```python
from build123d import *

# Parameters (mm, degrees)
SKETCH1_W               = 40
SKETCH1_H               = 55
SKETCH1_H_2             = 20
SKETCH1_R               = 2.5
BOSS_EXTRUDE1_DEPTH     = 10
SKETCH3_W               = 40
SKETCH3_H               = 10
BOSS_EXTRUDE2_DEPTH     = 40
SKETCH4_W               = 9
SKETCH4_H               = 3.5
BOSS_EXTRUDE3_DEPTH     = 40
SKETCH5_R               = 1.5
CUT_EXTRUDE1_DEPTH      = 3.5
SKETCH7_W               = 40
SKETCH7_H               = 3.5
BOSS_EXTRUDE4_DEPTH     = 80
SKETCH8_W               = 12
SKETCH8_H               = 40
BOSS_EXTRUDE5_DEPTH     = 35
SKETCH9_W               = 12
SKETCH9_H               = 23
CUT_EXTRUDE2_DEPTH      = 17
SKETCH10_R              = 1.7
CUT_EXTRUDE3_DEPTH      = 1
CUT_EXTRUDE3_DEPTH_BACK = 38.5
FILLET1_R               = 1
FILLET2_R               = 40


with BuildPart() as part:
    # Sketch1 → Boss-Extrude1 (new body)
    with BuildSketch(Plane(origin=(0, 0, 0), x_dir=(0, 0, -1), z_dir=(1, 0, 0))):
        with Locations((0, 27.5)):
            Rectangle(SKETCH1_W, SKETCH1_H)
        with Locations((0, -10)):
            Rectangle(SKETCH1_W, SKETCH1_H_2)
        with Locations((10, -10)):
            Circle(SKETCH1_R, mode=Mode.SUBTRACT)
        with Locations((-10, -10)):
            Circle(SKETCH1_R, mode=Mode.SUBTRACT)
    extrude(amount=BOSS_EXTRUDE1_DEPTH)

    # Sketch3 → Boss-Extrude2 (add)
    with BuildSketch(Plane.ZY):
        with Locations((0, 5)):
            Rectangle(SKETCH3_W, SKETCH3_H)
    extrude(amount=BOSS_EXTRUDE2_DEPTH)

    # Sketch4 → Boss-Extrude3 (add)
    with BuildSketch(Plane.ZY):
        with Locations((-15.5, 53.25)):
            Rectangle(SKETCH4_W, SKETCH4_H)
    boss_extrude3 = extrude(amount=BOSS_EXTRUDE3_DEPTH)

    # Sketch5 → Cut-Extrude1 (cut)
    with BuildSketch(Plane(origin=(0, 55, 0), x_dir=(1, 0, 0), z_dir=(0, 1, 0))):
        with Locations((-35, 15)):
            Circle(SKETCH5_R)
        with Locations((-4, 15)):
            Circle(SKETCH5_R)
    cut_extrude1 = extrude(amount=-CUT_EXTRUDE1_DEPTH, mode=Mode.SUBTRACT)

    # Mirror2: Boss-Extrude3, Cut-Extrude1 across plane
    add(boss_extrude3.mirror(Plane.XY))
    add(cut_extrude1.mirror(Plane.XY), mode=Mode.SUBTRACT)

    # Sketch7 → Boss-Extrude4 (add)
    with BuildSketch(Plane.XY.offset(20)):
        with Locations((-20, 53.25)):
            Rectangle(SKETCH7_W, SKETCH7_H)
        Polygon((10, 55), (0, 55), (0, 51.5), (0, 25), (10, 25), align=None)
    extrude(amount=BOSS_EXTRUDE4_DEPTH)

    # Sketch8 → Boss-Extrude5 (add)
    with BuildSketch(Plane(origin=(0, 55, 0), x_dir=(1, 0, 0), z_dir=(0, 1, 0))):
        with Locations((-20, -80)):
            Rectangle(SKETCH8_W, SKETCH8_H)
    extrude(amount=BOSS_EXTRUDE5_DEPTH)

    # Sketch9 → Cut-Extrude2 (cut)
    with BuildSketch(Plane(origin=(0, 0, 60), x_dir=(-1, 0, 0), z_dir=(0, 0, -1))):
        with Locations((20, 72.5)):
            Rectangle(SKETCH9_W, SKETCH9_H)
    extrude(amount=-CUT_EXTRUDE2_DEPTH, mode=Mode.SUBTRACT)

    # Sketch10 → Cut-Extrude3 (cut, two sides)
    with BuildSketch(Plane(origin=(0, 90, 0), x_dir=(1, 0, 0), z_dir=(0, 1, 0))) as cut_extrude3_sk:
        with Locations((-20, -68)):
            Circle(SKETCH10_R)
    extrude(amount=CUT_EXTRUDE3_DEPTH, mode=Mode.SUBTRACT)
    extrude(cut_extrude3_sk.sketch, amount=-CUT_EXTRUDE3_DEPTH_BACK, mode=Mode.SUBTRACT)

    # Fillet1
    fillet1_edges = [part.edges().sort_by_distance(p)[0] for p in [
        (-33, 55, 100),
        (-26, 55, 80),
        (-26, 87, 60),
        (-26, 72.5, 100),
        (-14, 55, 80),
        (-14, 72.5, 100),
        (-20, 55, 60),
        (-14, 87, 60),
        (-26, 90, 80),
        (-20, 90, 100),
        (-14, 90, 80),
        (-26, 58, 60),
        (-14, 58, 60),
        (-14, 72.5, 77),
        (-14, 61, 68.5),
        (-20, 84, 77),
        (-14, 84, 68.5),
        (-26, 72.5, 77),
        (-26, 84, 68.5),
        (-20, 61, 77),
        (-26, 61, 68.5),
        (-20, 51.5, 100),
        (0, 38.25, 100),
        (5, 25, 100),
        (10, 40, 100),
        (-2, 55, 100),
        (-40, 53.25, 100),
    ]]
    fillet(fillet1_edges, radius=FILLET1_R)

    # Fillet2
    fillet2_edges = [part.edges().sort_by_distance(p)[0] for p in [
        (5, 25, 20),
    ]]
    fillet(fillet2_edges, radius=FILLET2_R)


solid = part.part
```
Geometry check sheet. Reference: the model listing, model coordinates, mm. A direction names the side the tool comes from. Round coordinates to 2 decimals unless told otherwise and drop trailing zeros. Write each loop counter-clockwise with the first axis right and the second up, starting at its lowest first coordinate (ties: lowest second). Pieces come first, ordered by that corner, then holes. Notation, with made-up numbers: (10, 81) -> (19, 81) arc R7 cw to (19, 88) -> close; hole circle Ø11 at (27, 51). An arc over 180 degrees is marked (long way). Put each result on its own line as item: value.
1) Cross-section at C-C, the plane x = -20. Give the number of separate pieces and of enclosed holes in the cut face, plus the area to 3 significant figures.
Recorded:
separate pieces: 5
enclosed holes: 0
area: 1,750 mm2
2) Cross-section at A-A, the plane x = -9. Enter the section's corners in (y, z).
Recorded:
outline: (0, -20) -> (10, -20) -> (10, 28.78) arc R40 cw to (0, 22.92) -> close; (51.5, -20) -> (55, -20) -> (55, -11) -> (51.5, -11) -> close; (51.5, 11) -> (55, 11) -> (55, 99) arc R1 ccw to (54, 100) -> (52.5, 100) arc R1 ccw to (51.5, 99) -> close
3) Access from +Z, -Z, +X, -X, +Y, -Y to the whole of each face (thin tool, end or side, straight path). Record for faces 5 (the face through (-36.2, 53.3, 14.1)), 6 (the face through (-20, 10, 4)), 7 (the face through (5, 25, 79)), 8 (the face through (-20, 58, 60)), 9 (the face through (-20, 73, 77)).
Recorded:
face 5: +Y
face 6: +Z, -Z, -X
face 7: +Z, +X, -X, -Y
face 8: -Z, +X, -X, +Y
face 9: -Z, +X, -X
4) Cross-section at D-D, the plane z = 3. Enter the section's corners in (x, y), plus the area to 3 significant figures.
Recorded:
outline: (-40, 0) -> (0, 0) -> (0, -20) -> (10, -20) -> (10, 55) -> (0, 55) -> (0, 10) -> (-40, 10) -> close
area: 1,150 mm2
5) Thickness scan on probe 1 along X at (y, z) = (52, -15); probe 2 along X at (y, z) = (88, 68); probe 3 along Z at (x, y) = (-35, 52.5). Record the ranges inside material, lowest first. Write a range as from..to.
Recorded:
probe 1: x = -40..-36.5, -33.5..-5.5, -2.5..10
probe 2: x = -26..-21.7, -18.3..-14
probe 3: z = -20..-16.5, -13.5..-11, 11..13.5, 16.5..100
6) Cross-section at B-B, the plane z = -15. Enter the section's corners in (x, y).
Recorded:
outline: (-40, 0) -> (0, 0) -> (0, -20) -> (10, -20) -> (10, 55) -> (-2.5, 55) -> (-2.5, 51.5) -> (0, 51.5) -> (0, 10) -> (-40, 10) -> close; (-40, 51.5) -> (-36.5, 51.5) -> (-36.5, 55) -> (-40, 55) -> close; (-33.5, 51.5) -> (-5.5, 51.5) -> (-5.5, 55) -> (-33.5, 55) -> close
7) Depth check by flat-ended pin: P1, Ø10, axis at y = -5.5, z = 11.5, coming from the -X side; P2, Ø2.5, axis at x = -35, z = 15, coming from the -Y side; P3, Ø10, axis at x = -7.5, z = 38, coming from the +Y side. Enter the tip coordinate at first touch or a pass-through.
Recorded:
P1: stops at x = 0
P2: stops at y = 0
P3: stops at y = 55
8) Release check for a two-part mould opening along X. For faces 1 (the face through (-40, 5, 4)), 2 (the face through (-14, 72, 84)), 3 (the face through (-2.614, 53.274, 14.425)), 4 (the face through (4.93, -12.44, -9.46)) record: pulls with the +X half, pulls with the -X half, needs draft (parallel to the pull), parting line crosses it, or undercut.
Recorded:
face 1: pulls with the -X half
face 2: pulls with the +X half
face 3: undercut
face 4: needs draft
